The listing builds one solid part. Answer for the finished solid, in the listing's coordinates (mm). Face numbers are marked on the shaded views. A direction names the side the tool comes from. Give positions to 0.01 mm unless a question says otherwise; leave off trailing zeros. Write each loop counter-clockwise with the first axis right and the second up, starting at its lowest first coordinate (ties: lowest second). Pieces come first, ordered by that corner, then holes. Notation, with made-up numbers: M 61,-12 L 76,-12 A34 ccw 76,20 Z; hole C 17.25,50 d7. An arc over 180 degrees is marked long. Return JSON: item names as keys, results as strings.
from build123d import *

# Parameters (mm, degrees)
EXTRUDE_1_DEPTH      = 3.5
EXTRUDE_1_DEPTH_BACK = 5.5
SKETCH_1_R           = 6
SKETCH_2_R           = 4.75
EXTRUDE_2_DEPTH      = 11.5
SKETCH_3_R           = 4.25
CUT_EXTRUDE_1_DEPTH  = 11.5
SKETCH_4_W           = 14.6
SKETCH_4_H           = 12.5
EXTRUDE_3_DEPTH      = 14.2
SKETCH_5_R           = 1.25
EXTRUDE_4_DEPTH      = 1.5
CUT_EXTRUDE_2_DEPTH  = 9


with BuildPart() as part:
    # 草圖1 → 填料-伸長1 (new, two sides: drawn at the far end of the back side and taken through both)
    with BuildSketch(Plane.XY.offset(-EXTRUDE_1_DEPTH_BACK)):
        with Locations((-29.340909091, 31.5)):
            Circle(SKETCH_1_R)
    extrude(amount=EXTRUDE_1_DEPTH + EXTRUDE_1_DEPTH_BACK)

    # 草圖2 → 填料-伸長2 (add)
    with BuildSketch(Plane(origin=(0, 0, -5.5), x_dir=(-1, 0, 0), z_dir=(0, 0, -1))):
        with Locations((29.340909091, 31.5)):
            Circle(SKETCH_2_R)
    extrude(amount=EXTRUDE_2_DEPTH)

    # 草圖3 → 除料-伸長1 (cut)
    with BuildSketch(Plane(origin=(0, 0, -17), x_dir=(-1, 0, 0), z_dir=(0, 0, -1))):
        with Locations((29.340909091, 31.5)):
            Circle(SKETCH_3_R)
    extrude(amount=-CUT_EXTRUDE_1_DEPTH, mode=Mode.SUBTRACT)

    # 草圖4 → 填料-伸長3 (add)
    with BuildSketch(Plane.XY.offset(3.5)):
        with Locations((-29.340909091, 31.35)):
            Rectangle(SKETCH_4_W, SKETCH_4_H)
    extrude(amount=EXTRUDE_3_DEPTH)

    # 草圖5 → 填料-伸長4 (add)
    with BuildSketch(Plane.XZ.offset(-25.1)):
        with BuildLine():
            Line((-17.240909091, 5.697422491), (-46.240909091, 5.697422491))
            ThreePointArc((-46.240909091, 5.697422491), (-47.301569263, 6.136762319), (-47.740909091, 7.197422491))
            Line((-47.740909091, 7.197422491), (-47.740909091, 50.697422491))
            ThreePointArc((-47.740909091, 50.697422491), (-47.301569263, 51.758082663), (-46.240909091, 52.197422491))
            Line((-46.240909091, 52.197422491), (-17.240909091, 52.197422491))
            ThreePointArc((-17.240909091, 52.197422491), (-16.180248919, 51.758082663), (-15.740909091, 50.697422491))
            Line((-15.740909091, 50.697422491), (-15.740909091, 7.197422491))
            ThreePointArc((-15.740909091, 7.197422491), (-16.180248919, 6.136762319), (-17.240909091, 5.697422491))
        make_face()
        with Locations(Location((-17.740909091, 50.197422491, 0), (0, 0, 270))):
            Circle(SKETCH_5_R, mode=Mode.SUBTRACT)
        with Locations(Location((-45.740909091, 50.197422491, 0), (0, 0, 270))):
            Circle(SKETCH_5_R, mode=Mode.SUBTRACT)
    extrude(amount=EXTRUDE_4_DEPTH)

    # 草圖6 → 除料-伸長2 (cut)
    with BuildSketch(Plane(origin=(0, 0, -5.5), x_dir=(-1, 0, 0), z_dir=(0, 0, -1))):
        with BuildLine():
            Line((26.942993329, 26), (31.738824853, 26))
            ThreePointArc((31.738824853, 26), (29.340909091, 25.5), (26.942993329, 26))
        make_face()
        with BuildLine():
            Line((23.840909091, 29.102084238), (23.840909091, 33.897915762))
            ThreePointArc((23.840909091, 33.897915762), (23.340909091, 31.5), (23.840909091, 29.102084238))
        make_face()
        with BuildLine():
            Line((26.942993329, 37), (31.738824853, 37))
            ThreePointArc((31.738824853, 37), (29.340909091, 37.5), (26.942993329, 37))
        make_face()
        with BuildLine():
            Line((34.840909091, 29.102084238), (34.840909091, 33.897915762))
            ThreePointArc((34.840909091, 33.897915762), (35.340909091, 31.5), (34.840909091, 29.102084238))
        make_face()
    extrude(amount=-CUT_EXTRUDE_2_DEPTH, mode=Mode.SUBTRACT)


solid = part.part
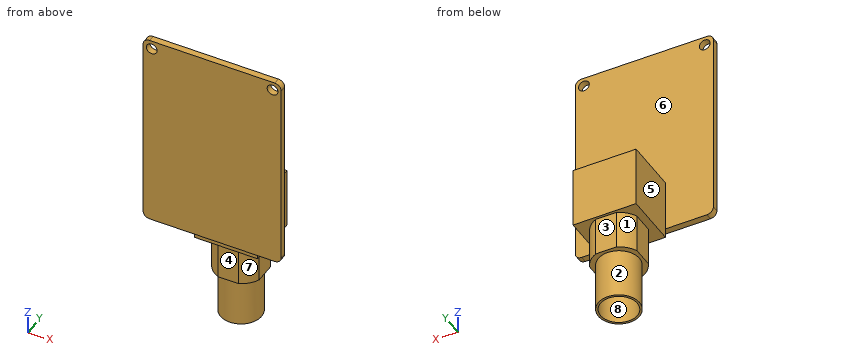
Item 1: A cutting plane is placed at B-B, the plane y = 31.5. Write down the section's boundary in (x, z).
Geometry results:
{"outline": "M -36.64,3.5 L -34.84,3.5 L -34.84,-5.5 L -34.09,-5.5 L -34.09,-17 L -33.59,-17 L -33.59,-5.5 L -25.09,-5.5 L -25.09,-17 L -24.59,-17 L -24.59,-5.5 L -23.84,-5.5 L -23.84,3.5 L -22.04,3.5 L -22.04,17.7 L -36.64,17.7 Z"}
Item 2: Given pin 1 Ø2.5 at (x, y) = (-29, 31) entering from -Z; pin 2 Ø1.5 at (x, z) = (-45.74, 50.2) entering from +Y; pin 3 Ø2 at (x, z) = (-40.5, 22) entering from +Y; pin 4 Ø6 at (y, z) = (28.5, 4.5) entering from -X, each flat-ended and moving along its own axis, determine where each tip first touches the part or whether it passes through.
Geometry results:
{"pin 1": "stops at z = -5.5", "pin 2": "passes through", "pin 3": "stops at y = 25.1", "pin 4": "stops at x = -36.64"}
Item 3: Which of the six approach directions +Z, -Z, +X, -X, +Y, -Y give full straight-line access (tool end or side, diameter ignored) to the marked faces 1, 2, 3 and 4?
Geometry results:
{"face 1": "-Z, -X, +Y", "face 2": "-Z", "face 3": "-Z, +X, -X, +Y", "face 4": "-Z, +X, -X, -Y"}
Item 4: Determine the mould class of the marked faces 5, 6, 7 and 8 for opening direction X: +X half, -X half, draft (parallel to the pull), parting line (faces both ways), or undercut.
Geometry results:
{"face 5": "-X half", "face 6": "draft", "face 7": "+X half", "face 8": "undercut"}
Item 5: A cutting plane is placed at A-A, the plane x = -36. Write down the section's boundary in (y, z), plus the area to 3 significant figures.
Geometry results:
{"outline": "M 23.6,5.7 L 25.1,5.7 L 25.1,3.5 L 37.6,3.5 L 37.6,17.7 L 25.1,17.7 L 25.1,52.2 L 23.6,52.2 Z", "area": "247 mm2"}
Item 6: A cutting plane is placed at D-D, the plane x = -28. Write down the section's boundary in (y, z).
Geometry results:
{"outline": "M 23.6,5.7 L 25.1,5.7 L 25.1,3.5 L 26,3.5 L 26,-5.5 L 26.94,-5.5 L 26.94,-17 L 27.47,-17 L 27.47,-5.5 L 35.53,-5.5 L 35.53,-17 L 36.06,-17 L 36.06,-5.5 L 37,-5.5 L 37,3.5 L 37.6,3.5 L 37.6,17.7 L 25.1,17.7 L 25.1,52.2 L 23.6,52.2 Z"}
Item 7: A cutting plane is placed at C-C, the plane z = 24. Write down the section's boundary in (x, y).
Geometry results:
{"outline": "M -47.74,23.6 L -15.74,23.6 L -15.74,25.1 L -47.74,25.1 Z"}
Item 8: Find the intervals of material crossed by line 1 (Y direction, x = -29, z = -10); line 2 (X direction, y = 27.5, z = 9); line 3 (Z direction, x = -22.5, y = 25.75), in increasing order.
Geometry results:
{"line 1": "y = 26.76 to 27.26, 35.74 to 36.24", "line 2": "x = -36.64 to -22.04", "line 3": "z = 3.5 to 17.7"}
